from build123d import *

# Parameters (mm, degrees)
SKETCH_1_W          = 15
SKETCH_1_H          = 10
EXTRUDE_1_DEPTH     = 10
SKETCH_1_3_W        = 15
SKETCH_1_3_H        = 10
EXTRUDE_2_DEPTH     = 20
CUT_EXTRUDE_1_DEPTH = 20


with BuildPart() as part:
    # Sketch 1 → Extrude 1 (new body)
    with BuildSketch(Plane(origin=(0, 0, 0), x_dir=(1, 0, 0), z_dir=(0, 1, 0))):
        with BuildLine():
            Line((-12.5, 10), (-12.5, -10))
            ThreePointArc((-12.5, -10), (-5.428932188, -7.071067812), (-2.5, 0))
            Line((-2.5, 0), (-2.5, 10))
            Line((-2.5, 10), (-12.5, 10))
        make_face()
        with BuildLine():
            ThreePointArc((-2.5, 0), (-5.428932188, -7.071067812), (-12.5, -10))
            Line((-12.5, -10), (-2.5, -10))
            Line((-2.5, -10), (12.5, -10))
            Line((12.5, -10), (12.5, 0))
            Line((12.5, 0), (-2.5, 0))
        make_face()
        with Locations((5, 5)):
            Rectangle(SKETCH_1_W, SKETCH_1_H)
    extrude(amount=EXTRUDE_1_DEPTH)

    # Sketch 1_3 → Extrude 2 (add)
    with BuildSketch(Plane(origin=(0, 0, 0), x_dir=(1, 0, 0), z_dir=(0, 1, 0))):
        with BuildLine():
            Line((-12.5, 10), (-12.5, -10))
            ThreePointArc((-12.5, -10), (-5.428932188, -7.071067812), (-2.5, 0))
            Line((-2.5, 0), (-2.5, 10))
            Line((-2.5, 10), (-12.5, 10))
        make_face()
        with Locations((5, 5)):
            Rectangle(SKETCH_1_3_W, SKETCH_1_3_H)
    extrude(amount=EXTRUDE_2_DEPTH)

    # Sketch 2 → Cut-Extrude 1 (cut)
    with BuildSketch(Plane.XY):
        Polygon((-2.5, 20), (12.5, 10), (12.5, 20), align=None)
    extrude(amount=-CUT_EXTRUDE_1_DEPTH, mode=Mode.SUBTRACT)


solid = part.part
Source: CAD feature listing. Evaluate the final solid. Frame: model axes, mm. A direction names the side the tool comes from. Round coordinates to 2 decimals unless told otherwise and drop trailing zeros. Loops run counter-clockwise (first coordinate to the right, second up) from the corner with the lowest first, then second, coordinate; pieces in that order, holes last. Notation, with made-up numbers: M 46.5,-8.5 L 104.5,-8.5 A18 ccw 104.5,1.5 Z; hole C 83,45 d6. An arc over 180 degrees is marked long. Return JSON: item names as keys, results as strings. Group by question number.
1. Reachability of faces 1 (the face through (12.5, 5, 0)), 2 (the face through (3, 14, 0)) from +Z, -Z, +X, -X, +Y, -Y: full face, straight path, thin tool, end or side. Return the list, or none.
2. Pin query (flat end, axial travel): pin 1 (5 mm diameter, centred on x = -4, z = 0.5, fed in from -Y). Return the tip coordinate at first contact, or that it passes through.
3. Material intervals for line 1 along Z through (x, y) = (2.5, 13.25); line 2 along Y through (x, z) = (5, 5.25); line 3 along Y through (x, z) = (5.5, -1.25), sorted ascending. Write a range as from..to.
4. Section query A-A on z = -0.75. Output: boundary loops of the cut face in (x, y).
5. Mould query, pull axis Y, two halves, no side actions, for faces 3 (the face through (0, 8, -10)), 4 (the face through (0, 0, 0)), 5 (the face through (3, 10, 5)). Classes: released by +Y, released by -Y, zero draft, split by the parting line, or undercut.
6. Section query C-C on y = 14.75. Output: boundary loops of the cut face in (x, z) (3 decimals), and give its area (3 significant figures).
7. Section query D-D on x = 6.75. Output: boundary loops of the cut face in (y, z).
8. Section query B-B on x = 2.5. Output: boundary loops of the cut face in (y, z).
Checks:
{
 "1": {"face 1": "+Z, -Z, +X, +Y, -Y", "face 2": "+Z, +X, +Y"},
 "2": {"pin 1": "stops at y = 0"},
 "3": {"line 1": "z = -10..0", "line 2": "y = 0..10", "line 3": "y = 0..14.67"},
 "4": {"outline": "M -12.5,0 L 12.5,0 L 12.5,10 L -2.5,20 L -12.5,20 Z"},
 "5": {"face 3": "zero draft", "face 4": "released by -Y", "face 5": "released by +Y"},
 "6": {"outline": "M -12.5,-10 L 5.375,-10 L 5.375,0 L -2.5,0 A10 ccw -12.5,10 Z", "area": "257 mm²"},
 "7": {"outline": "M 0,-10 L 13.83,-10 L 13.83,0 L 10,0 L 10,10 L 0,10 Z"},
 "8": {"outline": "M 0,-10 L 16.67,-10 L 16.67,0 L 10,0 L 10,10 L 0,10 Z"}
}
